Verification items for the finished model (mm, model axes). A direction names the side the tool comes from. Give positions to 0.01 mm unless a question says otherwise; leave off trailing zeros. Order: outer loops, then holes, each group sorted by start corner. A loop starts at its lowest first (then second) coordinate and runs counter-clockwise, first axis right, second up. Notation, with made-up numbers: (-29, 42.25) -> (-16, 42.25) arc R7 ccw to (-16, 53.25) -> close; hole circle Ø10 at (-24.5, 40). An arc over 180 degrees is marked (long way). One line per question, with ' | ' between items. Start each with the question number.
Q1. Mould release check, pull along X, two halves, no side actions. Record for faces 5 (the flat face through (5, 3, -23)), 6 (the cylindrical face through (41.4, 3.3, 5.93)), 7 (the flat face through (3, 3, -3)), 8 (the flat face through (28.75, 3, -14)): released by +X, released by -X, zero draft, split by the parting line, or undercut.
Q2. Access from +Z, -Z, +X, -X, +Y, -Y to the whole of each face (thin tool, end or side, straight path). Record for faces 1 (the flat face through (12.3, 3, -23)), 2 (the flat face through (24.25, 3, -14)), 3 (the flat face through (-2, 3, -42.75)), 4 (the flat face through (15, 3, 0)).
Q3. Section check A-A on z = -4. Record the cut outline in (x, y), plus the area to 3 significant figures.
Q4. Go/stop test with flat-tipped pins: pin 1 (3 mm diameter, centred on y = 4, z = -16, fed in from +X); pin 2 (3 mm diameter, centred on y = 3, z = -23.5, fed in from +X); pin 3 (2 mm diameter, centred on y = 3.5, z = -31, fed in from -X). Record where each tip stops, or that it passes through.
Q5. Material ranges on probe 1 along Z at (x, y) = (7, 2.5); probe 2 along Z at (x, y) = (-3, 3.75); probe 3 along X at (y, z) = (4.75, 1.5), recorded low to high. Write a range as [from, to].
Q6. Section check D-D on z = -44. Record the cut outline in (x, y).
Q7. Section check C-C on x = -2.5. Record the cut outline in (y, z).
Q8. Section check B-B on x = 4. Record the cut outline in (y, z).
Autodesk Inventor part; units mm, degrees
ref_plane "YZ Plane" through (0, 0, 0) normal (1, 0, 0) x (0, 1, 0)
ref_plane "XZ Plane" through (0, 0, 0) normal (0, 1, 0) x (-1, 0, 0)
ref_plane "XY Plane" through (0, 0, 0) normal (0, 0, 1) x (1, 0, 0)
sketch "Sketch1" plane through (0, 0, 0) normal (0, 1, 0) x (-1, 0, 0)
  line L0 (0, -51.7) -> (0, 0)
  line L1 (0, 0) -> (-50, 0)
  line L2 (-50, 0) -> (-50, -8)
  line L3 (-50, -8) -> (-6, -51.7)
  line L4 (-6, -51.7) -> (0, -51.7)
  dimension "d0" = 51.7
  dimension "d1" = 50
  dimension "d2" = 8
  dimension "d3" = 6
extrude "Extrusion1" add sketch "Sketch1" along normal blind 6.5
sketch "Sketch2" plane through (0, 6.5, 0) normal (0, 1, 0) x (1, 0, 0)
  line L0 (0, 0) -> (50, 0)
  line L1 (50, 0) -> (50, 8)
  line L2 (34, 0) -> (42, 0)
  line L3 (42, 0) -> (42, -4.5)
  line L4 (40, -6.5) -> (36, -6.5)
  line L5 (34, -4.5) -> (34, 0)
  arc A0 (34, -4.5) -> (36, -6.5) centre (36, -4.5) ccw
  arc A1 (40, -6.5) -> (42, -4.5) centre (40, -4.5) ccw
  dimension "d6" = 2
  dimension "d7" = 8
  dimension "d8" = 6.5
  dimension "d9" = 8
extrude "Extrusion2" add sketch "Sketch2" against normal blind 6.5
sketch "Sketch3" plane through (0, 6.5, 0) normal (0, 1, 0) x (1, 0, 0)
  line L0 (0, 0) -> (34, 0)
  line L1 (34, 0) -> (34, -4.5)
  line L2 (24.25, 16.3) -> (28.75, 16.3)
  line L3 (28.75, 0) -> (24.25, 0)
  line L4 (31.25, 12.3) -> (31.25, 5)
  line L5 (21.75, 5) -> (21.75, 12.3)
  line L6 (21.75, 12.3) -> (24.25, 12.3)
  line L7 (28.75, 12.3) -> (31.25, 12.3)
  line L8 (24.25, 0) -> (24.25, 5)
  line L9 (24.25, 12.3) -> (24.25, 16.3)
  line L10 (31.25, 5) -> (28.75, 5)
  line L11 (24.25, 5) -> (21.75, 5)
  line L12 (28.75, 16.3) -> (28.75, 12.3)
  line L13 (28.75, 5) -> (28.75, 0)
  point P0 (26.5, 16.3)
  dimension "d12" = 4.5
  dimension "d13" = 5
  dimension "d14" = 7.3
  dimension "d15" = 4
  dimension "d16" = 2.5
  dimension "d17" = 7.5
extrude "Extrusion3" cut sketch "Sketch3" against normal through all
sketch "Sketch4" plane through (0, 6.5, 0) normal (0, 1, 0) x (1, 0, 0)
  line L0 (0, 51.7) -> (0, 0)
  line L1 (0, 0) -> (24.25, 0)
  line L2 (16.3, 22) -> (16.3, 17.5)
  line L3 (0, 17.5) -> (0, 22)
  line L4 (5, 24.5) -> (12.3, 24.5)
  line L5 (12.3, 15) -> (5, 15)
  line L6 (0, 22) -> (5, 22)
  line L7 (12.3, 22) -> (16.3, 22)
  line L8 (16.3, 17.5) -> (12.3, 17.5)
  line L9 (5, 17.5) -> (0, 17.5)
  line L10 (5, 15) -> (5, 17.5)
  line L11 (5, 22) -> (5, 24.5)
  line L12 (12.3, 24.5) -> (12.3, 22)
  line L13 (12.3, 17.5) -> (12.3, 15)
  point P0 (16.3, 19.75)
  dimension "d20" = 4.5
  dimension "d21" = 5
  dimension "d22" = 4
  dimension "d23" = 7.3
  dimension "d24" = 19.75
  dimension "d25" = 2.5
extrude "Extrusion4" cut sketch "Sketch4" against normal through all
sketch "Sketch5" plane through (0, 6.5, 0) normal (0, 1, 0) x (1, 0, 0)
  line L0 (16.3, 22) -> (16.3, 17.5)
  line L1 (0, 51.7) -> (0, 22)
  line L2 (0, 42.75) -> (-4.5, 42.75)
  line L3 (-6.5, 40.75) -> (-6.5, 36.75)
  line L4 (-4.5, 34.75) -> (0, 34.75)
  line L5 (0, 34.75) -> (0, 42.75)
  arc A0 (-4.5, 42.75) -> (-6.5, 40.75) centre (-4.5, 40.75) ccw
  arc A1 (-6.5, 36.75) -> (-4.5, 34.75) centre (-4.5, 36.75) ccw
  point P0 (16.3, 19.75)
  dimension "d28" = 2
  dimension "d29" = 8
  dimension "d30" = 6.5
  dimension "d31" = 15
extrude "Extrusion5" add sketch "Sketch5" against normal blind 6.5
chamfer "Chamfer1" distance 6 angle 45 1 edges at (0, 3.25, 0)
properties part number "x_carryage_brace_top" material "Plywood, Finish"
Filled in:
1) face 5: undercut | face 6: released by +X | face 7: released by -X | face 8: undercut
2) face 1: +Y, -Y | face 2: +Z, +Y, -Y | face 3: -Z, -X, +Y, -Y | face 4: +Z, -X, +Y, -Y
3) outline: (2, 0) -> (24.25, 0) -> (24.25, 6.5) -> (2, 6.5) -> close; (28.75, 0) -> (50, 0) -> (50, 6.5) -> (28.75, 6.5) -> close | area: 283 mm²
4) pin 1: x = 43.46 | pin 2: x = 35.9 | pin 3: x = 0
5) probe 1: [-50.71, -24.5], [-15, 0] | probe 2: [-42.75, -34.75] | probe 3: [34, 42]
6) outline: (0, 0) -> (13.75, 0) -> (13.75, 6.5) -> (0, 6.5) -> close
7) outline: (0, -42.75) -> (6.5, -42.75) -> (6.5, -34.75) -> (0, -34.75) -> close
8) outline: (0, -51.7) -> (6.5, -51.7) -> (6.5, -22) -> (0, -22) -> close; (0, -17.5) -> (6.5, -17.5) -> (6.5, -2) -> (0, -2) -> close
